Geometry check sheet. Reference: the model listing, model coordinates, mm. A direction names the side the tool comes from. Give positions to 0.01 mm unless a question says otherwise; leave off trailing zeros. Write each loop counter-clockwise with the first axis right and the second up, starting at its lowest first coordinate (ties: lowest second). Pieces come first, ordered by that corner, then holes. Notation, with made-up numbers: M 52,18.5 L 97,18.5 A8 ccw 97,31.5 Z; hole C 43,32.5 d6. An arc over 180 degrees is marked long. One line per item, written item: value. Start each with the question number.
1. Cross-section at B-B on x = 6. Record the cut outline in (y, z).
2. Cross-section at D-D on x = 29.5. Record the cut outline in (y, z), then the cut area to 3 significant figures.
3. Cross-section at A-A on z = 4. Record the cut outline in (x, y).
4. Scan lines: line 1 (X direction, y = 1.5, z = -39); line 2 (Z direction, x = 32, y = 1.15); line 3 (Z direction, x = 55, y = 0.8). Record each from-to range of solid material in increasing order.
5. Cross-section at C-C on y = 0.95. Record the cut outline in (x, z), then the cut area to 3 significant figures.
6. Gauge pin test, flat ends, axial feed: pin 1 (0.8 mm diameter, centred on x = 17, y = 0.5, fed in from +Z); pin 2 (0.5 mm diameter, centred on y = 0.5, z = -15, fed in from -X); pin 3 (3 mm diameter, centred on x = 54.91, z = -18.32, fed in from +Y). Record the tip position at first contact, or that the pin passes through.
7. Tool access check on faces 1 (the face through (49, 1.588, -16)), 2 (the face through (45.474, 1, -16)). Record the directions out of +Z, -Z, +X, -X, +Y, -Y that give a thin tool (end or side, any length) a straight path to the whole face; none if there is none.
8. Release check for a two-part mould opening along X. For faces 3 (the face through (43.3, 0.78, -3.41)), 4 (the face through (55.97, 0.78, 4.54)), 5 (the face through (79.094, 0.783, 0.878)) record: pulls with the +X half, pulls with the -X half, needs draft (parallel to the pull), parting line crosses it, or undercut.
Autodesk Inventor part; units mm, degrees
ref_plane "YZ Plane" through (0, 0, 0) normal (1, 0, 0) x (0, 1, 0)
ref_plane "XZ Plane" through (0, 0, 0) normal (0, 1, 0) x (-1, 0, 0)
ref_plane "XY Plane" through (0, 0, 0) normal (0, 0, 1) x (1, 0, 0)
sketch "Sketch1" plane through (0, 0, 0) normal (0, 1, 0) x (-1, 0, 0)
  line L0 (-37.8542, -1.1176) -> (-32.7742, -1.1176)
  line L1 (-7.3742, -30.9118) -> (-37.8542, -30.9118)
  line L2 (-45.4742, -23.2918) -> (-45.4742, -8.7376)
  arc A0 (-37.8542, -1.1176) -> (-45.4742, -8.7376) centre (-37.8542, -8.7376) ccw
  arc A1 (-45.4742, -23.2918) -> (-37.8542, -30.9118) centre (-37.8542, -23.2918) ccw
  circle A2 centre (-72.8662, -0.3634) radius 2.3114
  circle A3 centre (-54.9057, -18.324) radius 2.3114
  circle A4 centre (-58.1742, 5.2324) radius 2.3114
  circle A5 centre (-32.7742, 5.2324) radius 2.3114
  circle A6 centre (-32.7742, -37.2618) radius 2.3114
  circle A7 centre (-7.3742, -37.2618) radius 2.3114
  arc A8 (-75.1264, 5.5707) -> (-77.3564, -4.8536) centre (-72.8662, -0.3634) ccw
  arc A9 (-32.7742, -43.6118) -> (-31.4271, -43.4673) centre (-32.7742, -37.2618) ccw
  arc A10 (-7.3742, -43.6118) -> (-7.3742, -30.9118) centre (-7.3742, -37.2618) ccw
  arc A11 (-32.7742, -1.1176) -> (-32.7742, 11.5824) centre (-32.7742, 5.2324) ccw
  arc A12 (-58.1742, 11.5824) -> (-60.4344, 11.1665) centre (-58.1742, 5.2324) ccw
  line L3 (-32.7742, 11.5824) -> (-58.1742, 11.5824)
  line L4 (-75.1264, 5.5707) -> (-60.4344, 11.1665)
  line L5 (-77.3564, -4.8536) -> (-42.3179, -39.8921)
  line L6 (-33.3376, -43.6118) -> (-7.3742, -43.6118)
  arc A13 (-42.3179, -39.8921) -> (-33.3376, -43.6118) centre (-33.3376, -30.9118) ccw
  line L7 (-37.8542, -1.1176) -> (-32.7742, -1.1176)
  point P0 (0, 0)
  point P1 (-45.4742, -30.9118)
  dimension "d2" = 7.62
  dimension "d20" = 12.7
  dimension "d21" = 29.7942
extrude "Extrusion1" add sketch "Sketch1" along normal blind 1.5875
properties part number "gusset-2-3.25-half"
Report:
1. outline: M 0,-43.46 L 1.59,-43.46 L 1.59,-39.12 L 0,-39.12 Z; M 0,-35.4 L 1.59,-35.4 L 1.59,-31.06 L 0,-31.06 Z
2. outline: M 0,-43.61 L 1.59,-43.61 L 1.59,-30.91 L 0,-30.91 Z; M 0,-0.21 L 1.59,-0.21 L 1.59,10.67 L 0,10.67 Z
2. area: 37.4 mm^2
3. outline: M 26.54,0 L 30.82,0 L 30.82,1.59 L 26.54,1.59 Z; M 34.73,0 L 56.22,0 L 56.22,1.59 L 34.73,1.59 Z; M 60.13,0 L 77.48,0 L 77.48,1.59 L 60.13,1.59 Z
4. line 1: x = 1.27 to 5.85, 8.9 to 31.25, 34.3 to 43.21
4. line 2: z = -43.61 to -39.44, -35.08 to -30.91, -1.07 to 3.05, 7.41 to 11.54
4. line 3: z = -27.21 to -20.63, -16.01 to 11.58
5. outline: M 7.37,-43.61 L 33.34,-43.61 A12.7 ccw 42.32,-39.89 L 77.36,-4.85 A6.35 ccw 75.13,5.57 L 60.43,11.17 A6.35 ccw 58.17,11.58 L 32.77,11.58 A6.35 ccw 32.77,-1.12 L 37.85,-1.12 A7.62 cw 45.47,-8.74 L 45.47,-23.29 A7.62 cw 37.85,-30.91 L 7.37,-30.91 A6.35 ccw Z; hole C 7.37,-37.26 d4.62; hole C 32.77,-37.26 d4.62; hole C 32.77,5.23 d4.62; hole C 54.91,-18.32 d4.62; hole C 58.17,5.23 d4.62; hole C 72.87,-0.36 d4.62
5. area: 1,650 mm^2
6. pin 1: stops at z = -30.91
6. pin 2: stops at x = 45.47
6. pin 3: passes through
7. face 1: +Z, -Z, +X, -X, +Y
7. face 2: -X, +Y, -Y
8. face 3: pulls with the -X half
8. face 4: undercut
8. face 5: pulls with the +X half
